Model file for the job. Use its own axes, mm. A direction names the side the tool comes from. Give positions to 0.01 mm unless a question says otherwise; leave off trailing zeros. Order: outer loops, then holes, each group sorted by start corner. A loop starts at its lowest first (then second) coordinate and runs counter-clockwise, first axis right, second up. Notation, with made-up numbers: M 25.25,26 L 33.25,26 A10 cw 33.25,35 Z; hole C 69,13.5 d1. An arc over 180 degrees is marked long. Return JSON: item names as keys, results as strings. Group by question number.
1. Two-plate mould, pull along X, no slides. Class faces 4 (the face through (-2, 1, 0)), 5 (the face through (1.336, -0.493, 0.786)), 6 (the face through (-1, 2.1, 1)): released by +X, released by -X, zero draft, split by the parting line, or undercut.
2. Slice it at C-C on z = -0.85. List the corners of the cut face in (x, y).
3. 3-axis set-ups, long thin cutter, end or side, ignore diameter. For faces 1 (the face through (1.35, -0.49, -0.76)), 2 (the face through (0.9, -0.49, 2.86)), 3 (the face through (-1, 0, 2)): which of +Z, -Z, +X, -X, +Y, -Y reach the whole face in a straight line?
4. Pin check, flat tips, straight feed: pin 1 (1.5 mm diameter, centred on x = 0, z = -1.5, fed in from -Y); pin 2 (1.3 mm diameter, centred on x = 0, z = 0, fed in from -Y); pin 3 (1 mm diameter, centred on x = -0.5, y = 1.5, fed in from +Z); pin 4 (1.5 mm diameter, centred on y = 2, z = -2, fed in from +X). Stop position of each tip, or through.
5. Slice it at D-D on x = -1.55. List the corners of the cut face in (y, z), then the cut area to 3 significant figures.
6. Wall check: probe 1 along X at (y, z) = (1.4, 0) (3 decimals); probe 2 along Y at (x, z) = (2.05, 1.8); probe 3 along Z at (x, y) = (-0.75, -0.55). Give the ranges that are in metal, low to high. Write a range as [from, to].
7. Slice it at B-B on y = -0.65. List the corners of the cut face in (x, z), then the cut area to 3 significant figures.
8. Slice it at A-A on x = 0. List the corners of the cut face in (y, z) (3 decimals).
from build123d import *

# Parameters (mm, degrees)
SKETCH1_R               = 2
BOSS_EXTRUDE1_DEPTH     = 2.1
SKETCH1_3_R             = 3
BOSS_EXTRUDE2_DEPTH     = 1
CUT_EXTRUDE1_DEPTH      = 5.733920151
CUT_EXTRUDE1_DEPTH_BACK = 5.733920151
SKETCH1_4_R             = 1.125


with BuildPart() as part:
    # Sketch1 → Boss-Extrude1 (new body)
    with BuildSketch(Plane(origin=(0, 0, 0), x_dir=(1, 0, 0), z_dir=(0, 1, 0))):
        with Locations(Location((0, 0, 0), (0, 0, 270))):
            Circle(SKETCH1_R)
    extrude(amount=BOSS_EXTRUDE1_DEPTH)

    # Sketch1_3 → Boss-Extrude2 (add)
    with BuildSketch(Plane(origin=(0, 0, 0), x_dir=(1, 0, 0), z_dir=(0, 1, 0))):
        with Locations(Location((0, 0, 0), (0, 0, 270))):
            Circle(SKETCH1_3_R)
        Polygon((0.894892917, -1.55), (1.789785834, 0), (0.894892917, 1.55), (-0.894892917, 1.55), (-1.789785834, 0), (-0.894892917, -1.55), align=None, mode=Mode.SUBTRACT)
    extrude(amount=-BOSS_EXTRUDE2_DEPTH)

    # Sketch1_4 → Cut-Extrude1 (cut, two sides: drawn at the far end of the back side and taken through both)
    with BuildSketch(Plane(origin=(0, 0, 0), x_dir=(1, 0, 0), z_dir=(0, 1, 0)).offset(-CUT_EXTRUDE1_DEPTH_BACK)):
        with Locations(Location((0, 0, 0), (0, 0, 270))):
            Circle(SKETCH1_4_R)
    extrude(amount=CUT_EXTRUDE1_DEPTH + CUT_EXTRUDE1_DEPTH_BACK, mode=Mode.SUBTRACT)


solid = part.part
Result:
{
 "1": {"face 4": "split by the parting line", "face 5": "undercut", "face 6": "zero draft"},
 "2": {"outline": "M -2.88,-1 L -1.3,-1 L -1.3,0 L -0.74,0 L -0.74,2.1 L -1.81,2.1 L -1.81,0 L -2.88,0 Z; M 0.74,0 L 1.3,0 L 1.3,-1 L 2.88,-1 L 2.88,0 L 1.81,0 L 1.81,2.1 L 0.74,2.1 Z"},
 "3": {"face 1": "-Y", "face 2": "+Y, -Y", "face 3": "+Y"},
 "4": {"pin 1": "stops at y = -1", "pin 2": "passes through", "pin 3": "stops at z = 2", "pin 4": "stops at x = 1.56"},
 "5": {"outline": "M -1,-2.57 L 0,-2.57 L 0,-1.26 L 2.1,-1.26 L 2.1,1.26 L 0,1.26 L 0,2.57 L -1,2.57 L -1,0.42 L 0,0.42 L 0,-0.42 L -1,-0.42 Z", "area": "9.61 mm2"},
 "6": {"probe 1": "x = [-2, -1.125], [1.125, 2]", "probe 2": "y = [-1, 0]", "probe 3": "z = [-2.9, -1.55], [1.55, 2.9]"},
 "7": {"outline": "C 0,0 d6; hole M -1.79,0 L -0.89,-1.55 L 0.89,-1.55 L 1.79,0 L 0.89,1.55 L -0.89,1.55 Z", "area": "20.0 mm2"},
 "8": {"outline": "M -1,-3 L 0,-3 L 0,-2 L 2.1,-2 L 2.1,-1.125 L 0,-1.125 L 0,-1.55 L -1,-1.55 Z; M -1,1.55 L 0,1.55 L 0,1.125 L 2.1,1.125 L 2.1,2 L 0,2 L 0,3 L -1,3 Z"}
}
